```python
from build123d import *

# Parameters (mm, degrees)
IZIM1_W                     = 63.5
IZIM1_H                     = 80
Y_KSEKLIK_EKSTR_ZYON1_DEPTH = 1.5
IZIM2_W                     = 63.5
IZIM2_H                     = 80
IZIM2_W_2                   = 60.5
IZIM2_H_2                   = 77
Y_KSEKLIK_EKSTR_ZYON2_DEPTH = 5.5
RADYUS1_R                   = 2
KES_EKSTR_ZYON2_DEPTH       = 0.5
IZIM8_W                     = 3
IZIM8_H                     = 3
Y_KSEKLIK_EKSTR_ZYON4_DEPTH = 5.5
IZIM9_R                     = 0.925
KES_EKSTR_ZYON4_DEPTH       = 5
IZIM10_W                    = 4
IZIM10_H                    = 8.3
KES_EKSTR_ZYON5_DEPTH       = 2
KES_EKSTR_ZYON6_DEPTH       = 1.5


with BuildPart() as part:
    # Çizim1 → Yükseklik-Ekstrüzyon1 (new body)
    with BuildSketch(Plane.XY):
        Rectangle(IZIM1_W, IZIM1_H)
    extrude(amount=Y_KSEKLIK_EKSTR_ZYON1_DEPTH)

    # Çizim2 → Yükseklik-Ekstrüzyon2 (add)
    with BuildSketch(Plane.XY.offset(1.5)):
        Rectangle(IZIM2_W, IZIM2_H)
        Rectangle(IZIM2_W_2, IZIM2_H_2, mode=Mode.SUBTRACT)
    extrude(amount=Y_KSEKLIK_EKSTR_ZYON2_DEPTH)

    # Radyus1
    radyus1_edges = [part.edges().sort_by_distance(p)[0] for p in [
        (31.75, -40, 3.5),
        (-31.75, -40, 3.5),
        (-31.75, 40, 3.5),
        (31.75, 40, 3.5),
    ]]
    fillet(radyus1_edges, radius=RADYUS1_R)

    # Çizim6 → Kes-Ekstrüzyon2 (cut)
    with BuildSketch(Plane(origin=(0, 0, 0), x_dir=(-1, 0, 0), z_dir=(0, 0, -1))):
        with BuildLine():
            Line((-3.535533906, 18.535533906), (-5.303300859, 20.303300859))
            ThreePointArc((-5.303300859, 20.303300859), (-7.5, 15), (-5.303300859, 9.696699141))
            Line((-5.303300859, 9.696699141), (-3.535533906, 11.464466094))
            ThreePointArc((-3.535533906, 11.464466094), (-5, 15), (-3.535533906, 18.535533906))
        make_face()
        with BuildLine():
            Line((3.535533906, 18.535533906), (5.303300859, 20.303300859))
            ThreePointArc((5.303300859, 20.303300859), (7.5, 15), (5.303300859, 9.696699141))
            Line((5.303300859, 9.696699141), (3.535533906, 11.464466094))
            ThreePointArc((3.535533906, 11.464466094), (5, 15), (3.535533906, 18.535533906))
        make_face()
        with BuildLine():
            Line((-8.838834765, 23.838834765), (-10.606601718, 25.606601718))
            ThreePointArc((-10.606601718, 25.606601718), (-15, 15), (-10.606601718, 4.393398282))
            Line((-10.606601718, 4.393398282), (-8.838834765, 6.161165235))
            ThreePointArc((-8.838834765, 6.161165235), (-12.5, 15), (-8.838834765, 23.838834765))
        make_face()
        with BuildLine():
            Line((-14.142135624, 29.142135624), (-15.909902577, 30.909902577))
            ThreePointArc((-15.909902577, 30.909902577), (-22.5, 15), (-15.909902577, -0.909902577))
            Line((-15.909902577, -0.909902577), (-14.142135624, 0.857864376))
            ThreePointArc((-14.142135624, 0.857864376), (-20, 15), (-14.142135624, 29.142135624))
        make_face()
        with BuildLine():
            Line((8.838834765, 23.838834765), (10.606601718, 25.606601718))
            ThreePointArc((10.606601718, 25.606601718), (15, 15), (10.606601718, 4.393398282))
            Line((10.606601718, 4.393398282), (8.838834765, 6.161165235))
            ThreePointArc((8.838834765, 6.161165235), (12.5, 15), (8.838834765, 23.838834765))
        make_face()
        with BuildLine():
            Line((14.142135624, 29.142135624), (15.909902577, 30.909902577))
            ThreePointArc((15.909902577, 30.909902577), (22.5, 15), (15.909902577, -0.909902577))
            Line((15.909902577, -0.909902577), (14.142135624, 0.857864376))
            ThreePointArc((14.142135624, 0.857864376), (20, 15), (14.142135624, 29.142135624))
        make_face()
    extrude(amount=-KES_EKSTR_ZYON2_DEPTH, mode=Mode.SUBTRACT)

    # Çizim8 → Yükseklik-Ekstrüzyon4 (add)
    with BuildSketch(Plane.XY.offset(1.5)):
        with Locations((-28.75, 37)):
            Rectangle(IZIM8_W, IZIM8_H)
        with Locations((28.75, 37)):
            Rectangle(IZIM8_W, IZIM8_H)
        with Locations((28.75, -37)):
            Rectangle(IZIM8_W, IZIM8_H)
        with Locations((-28.75, -37)):
            Rectangle(IZIM8_W, IZIM8_H)
    extrude(amount=Y_KSEKLIK_EKSTR_ZYON4_DEPTH)

    # Çizim9 → Kes-Ekstrüzyon4 (cut)
    with BuildSketch(Plane.XY.offset(7)):
        with Locations((-29.5, 37.75)):
            Circle(IZIM9_R)
        with Locations(Location((29.5, 37.75, 0), (0, 0, 180))):
            Circle(IZIM9_R)
        with Locations((29.5, -37.75)):
            Circle(IZIM9_R)
        with Locations(Location((-29.5, -37.75, 0), (0, 0, 180))):
            Circle(IZIM9_R)
    extrude(amount=-KES_EKSTR_ZYON4_DEPTH, mode=Mode.SUBTRACT)

    # Çizim10 → Kes-Ekstrüzyon5 (cut)
    with BuildSketch(Plane(origin=(31.75, 0, 0), x_dir=(0, 0, -1), z_dir=(1, 0, 0))):
        with Locations((-5, -19.45)):
            Rectangle(IZIM10_W, IZIM10_H)
    extrude(amount=-KES_EKSTR_ZYON5_DEPTH, mode=Mode.SUBTRACT)

    # Çizim11 → Kes-Ekstrüzyon6 (cut)
    with BuildSketch(Plane.XY.offset(1.5)):
        with BuildLine():
            Line((-22.25, -36), (-19.25, -36))
            ThreePointArc((-19.25, -36), (-18.257492443, -36.877816736), (-19.007464375, -37.9701425))
            Line((-19.007464375, -37.9701425), (-22.25, -38))
            ThreePointArc((-22.25, -38), (-23.25, -37), (-22.25, -36))
        make_face()
        with BuildLine():
            Line((19.25, -36), (22.25, -36))
            ThreePointArc((22.25, -36), (23.25, -37), (22.25, -38))
            Line((22.25, -38), (19.25, -38))
            ThreePointArc((19.25, -38), (18.25, -37), (19.25, -36))
        make_face()
    extrude(amount=-KES_EKSTR_ZYON6_DEPTH, mode=Mode.SUBTRACT)


solid = part.part
```
The listing builds one solid part. Answer for the finished solid, in the listing's coordinates (mm). A direction names the side the tool comes from. Round coordinates to 2 decimals unless told otherwise and drop trailing zeros. Loops run counter-clockwise (first coordinate to the right, second up) from the corner with the lowest first, then second, coordinate; pieces in that order, holes last. Notation, with made-up numbers: (53.25, 44) - (77.25, 44) arc R28 ccw to (77.25, 66) - close; hole circle Ø8 at (-36, -37). An arc over 180 degrees is marked (long way). Return JSON: item names as keys, results as strings. Group by question number.
1. Which of the six approach directions +Z, -Z, +X, -X, +Y, -Y give full straight-line access (tool end or side, diameter ignored) to faces 4 (the flat face through (15, 0, 0.2)), 5 (the cylindrical face through (31.15, -39.43, 3.55)), 6 (the flat face through (-29, 35.5, 4))?
2. The part is cut by section D-D on x = -11.5. Determine the outline of the cut face in (y, z), then the cut area to 3 significant figures.
3. The part is cut by section C-C on x = -24.5. Determine the outline of the cut face in (y, z), then the cut area to 4 significant figures.
4. The mould has two halves that part along Y. Classify faces 1 (the flat face through (0, -40, 3)), 2 (the flat face through (-9.7, 24.7, 0.2)), 3 (the flat face through (0, 1, 0)): pulls with the +Y half, pulls with the -Y half, needs draft (parallel to the pull), parting line crosses it, or undercut.
5. Consider probe 1 along X at (y, z) = (-37.75, 5.85) (3 decimals); probe 2 along Y at (x, z) = (-29.5, 5) (3 decimals); probe 3 along X at (y, z) = (33, 4). Determine where each line is inside the solid, lowest interval first.
6. The part is cut by section A-A on z = 4.75. Determine the outline of the cut face in (x, y) (3 decimals), then the cut area to 3 significant figures.
7. The part is cut by section B-B on y = -30. Determine the outline of the cut face in (x, z).
8. This flat-tipped pin is pushed along its axis until it touches: P1, Ø1.6, axis at x = 31, z = 4.5, coming from the -Y side. Where does it stop, or does it pass through?
Resolved:
{
 "1": {"face 4": "-Z", "face 5": "+Z, -Z, +X, -Y", "face 6": "+Z"},
 "2": {"outline": "(-40, 0) - (5.37, 0) - (5.37, 0.5) - (10.1, 0.5) - (10.1, 0) - (19.9, 0) - (19.9, 0.5) - (24.63, 0.5) - (24.63, 0) - (40, 0) - (40, 7) - (38.5, 7) - (38.5, 1.5) - (-38.5, 1.5) - (-38.5, 7) - (-40, 7) - close", "area": "132 mm²"},
 "3": {"outline": "(-40, 0) - (40, 0) - (40, 7) - (38.5, 7) - (38.5, 1.5) - (-38.5, 1.5) - (-38.5, 7) - (-40, 7) - close", "area": "136.5 mm²"},
 "4": {"face 1": "pulls with the -Y half", "face 2": "undercut", "face 3": "needs draft"},
 "5": {"probe 1": "x = -31.75 to -30.425, -28.575 to -27.25, 27.25 to 28.575, 30.425 to 31.75", "probe 2": "y = -40 to -38.675, -36.825 to -35.5, 35.5 to 36.825, 38.675 to 40", "probe 3": "x = -31.75 to -30.25, 30.25 to 31.75"},
 "6": {"outline": "(-31.75, -38) arc R2 ccw to (-29.75, -40) - (29.75, -40) arc R2 ccw to (31.75, -38) - (31.75, -23.6) - (30.25, -23.6) - (30.25, -35.5) - (27.25, -35.5) - (27.25, -38.5) - (-27.25, -38.5) - (-27.25, -35.5) - (-30.25, -35.5) - (-30.25, 35.5) - (-27.25, 35.5) - (-27.25, 38.5) - (27.25, 38.5) - (27.25, 35.5) - (30.25, 35.5) - (30.25, -15.3) - (31.75, -15.3) - (31.75, 38) arc R2 ccw to (29.75, 40) - (-29.75, 40) arc R2 ccw to (-31.75, 38) - close; hole circle Ø1.85 at (-29.5, -37.75); hole circle Ø1.85 at (-29.5, 37.75); hole circle Ø1.85 at (29.5, -37.75); hole circle Ø1.85 at (29.5, 37.75)", "area": "431 mm²"},
 "7": {"outline": "(-31.75, 0) - (31.75, 0) - (31.75, 7) - (30.25, 7) - (30.25, 1.5) - (-30.25, 1.5) - (-30.25, 7) - (-31.75, 7) - close"},
 "8": {"P1": "stops at y = -39.95"}
}
